Check sheet for the modelled part. Datum: model origin and axes. Units: mm. A direction names the side the tool comes from. Give positions to 0.01 mm unless a question says otherwise; leave off trailing zeros. Order: outer loops, then holes, each group sorted by start corner. A loop starts at its lowest first (then second) coordinate and runs counter-clockwise, first axis right, second up. Notation, with made-up numbers: (-28.5, 88.25) -> (-19.5, 88.25) arc R32 ccw to (-19.5, 127.25) -> close; hole circle Ø8 at (-22, 42.5). An arc over 180 degrees is marked (long way). One line per question, with ' | ' between items.
Autodesk Inventor part; units mm, degrees
ref_plane "YZ Plane" through (0, 0, 0) normal (1, 0, 0) x (0, 1, 0)
ref_plane "XZ Plane" through (0, 0, 0) normal (0, 1, 0) x (-1, 0, 0)
ref_plane "XY Plane" through (0, 0, 0) normal (0, 0, 1) x (1, 0, 0)
sketch "草圖1" plane through (0, 0, 0) normal (0, 1, 0) x (-1, 0, 0)
  line L0 (12, 16.5) -> (-12, 16.5)
  line L1 (-12, -16.5) -> (12, -16.5)
  line L2 (12, -16.5) -> (12, 16.5)
  line L3 (6.1, 11.4) -> (-6.1, 11.4)
  line L4 (-6.1, 11.4) -> (-6.1, -11.4)
  line L5 (-6.1, -11.4) -> (6.1, -11.4)
  line L6 (6.1, -11.4) -> (6.1, 11.4)
  circle A0 centre (8.5, 13.7) radius 1.5
  line L7 (12, 6) -> (9, 6)
  line L8 (9, 6) -> (9, -6)
  line L9 (9, -6) -> (12, -6)
  line L10 (12, -6) -> (12, 6)
  line L11 (0, -23.1) -> (0, 23.1)
  line L12 (16.8, 0) -> (-16.8, 0)
  circle A1 centre (8.5, -13.7) radius 1.5
  circle A2 centre (-8.5, 13.7) radius 1.5
  line L13 (-12, 6) -> (-9, 6)
  line L14 (-9, 6) -> (-9, -6)
  line L15 (-9, -6) -> (-12, -6)
  circle A3 centre (-8.5, -13.7) radius 1.5
  line L16 (-12, 16.5) -> (-12, 6)
  line L17 (-12, -6) -> (-12, -16.5)
  point P0 (0, 0)
  dimension "d0" = 16.5
  dimension "d1" = 33
  dimension "d2" = 24
  dimension "d4" = 12.2
  dimension "d5" = 22.8
  dimension "d6" = 6.1
  dimension "d7" = 11.4
  dimension "d8" = 3
  dimension "d9" = 3.5
  dimension "d10" = 2.8
  dimension "d11" = 12
  dimension "d12" = 3
  dimension "d13" = 6
extrude "擠出1" add sketch "草圖1" along normal mid plane 3 contours L2 L7 L8 L12 L6 L3 L11 L0 | L11 L3 L4 L12 L14 L13 L16 L0 | L2 L1 L11 L5 L6 L12 L8 L9 | L4 L5 L11 L1 L17 L15 L14 L12
fillet "圓角1" radius 3 4 edges at (12, 0, 16.5) (-12, 0, 16.5) (-12, 0, -16.5) (12, 0, -16.5)
properties part number "板子7"
Q1. Section check A-A (x = -2.75). Enter the section's corners in (y, z).
Result sheet:
outline: (-1.5, -16.5) -> (1.5, -16.5) -> (1.5, -11.4) -> (-1.5, -11.4) -> close; (-1.5, 11.4) -> (1.5, 11.4) -> (1.5, 16.5) -> (-1.5, 16.5) -> close
Q2. Depth check by flat-ended pin: pin 1 Ø0.9 at (x, y) = (11, 0.5) entering from +Z; pin 2 Ø1 at (y, z) = (0, 2) entering from -X; pin 3 Ø0.9 at (x, y) = (10.5, 0.5) entering from -Z. Enter the tip coordinate at first touch or a pass-through.
Result sheet:
pin 1: stops at z = 16.07 | pin 2: stops at x = -9 | pin 3: stops at z = -16.31
Q3. Section check B-B (z = -4). Enter the section's corners in (x, y), and give its area (3 significant figures).
Result sheet:
outline: (-9, -1.5) -> (-6.1, -1.5) -> (-6.1, 1.5) -> (-9, 1.5) -> close; (6.1, -1.5) -> (9, -1.5) -> (9, 1.5) -> (6.1, 1.5) -> close | area: 17.4 mm2
Q4. Thickness scan on line 1 (Z direction, x = 8.5, y = 0); line 2 (Z direction, x = -9.75, y = 0.4); line 3 (X direction, y = -0.75, z = -12.5). Record the ranges inside material, lowest first.
Result sheet:
line 1: z = -16.5 to -15.2, -12.2 to 12.2, 15.2 to 16.5 | line 2: z = -16.4 to -14.53, -12.87 to -6, 6 to 12.87, 14.53 to 16.4 | line 3: x = -12 to -9.4, -7.6 to 7.6, 9.4 to 12
Q5. Section check D-D (x = -8.5). Enter the section's corners in (y, z), and give its area (3 significant figures).
Result sheet:
outline: (-1.5, -16.5) -> (1.5, -16.5) -> (1.5, -15.2) -> (-1.5, -15.2) -> close; (-1.5, -12.2) -> (1.5, -12.2) -> (1.5, 12.2) -> (-1.5, 12.2) -> close; (-1.5, 15.2) -> (1.5, 15.2) -> (1.5, 16.5) -> (-1.5, 16.5) -> close | area: 81.0 mm2
Q6. Section check C-C (y = -0.95). Enter the section's corners in (x, z), and give its area (3 significant figures).
Result sheet:
outline: (-12, -13.5) arc R3 ccw to (-9, -16.5) -> (9, -16.5) arc R3 ccw to (12, -13.5) -> (12, -6) -> (9, -6) -> (9, 6) -> (12, 6) -> (12, 13.5) arc R3 ccw to (9, 16.5) -> (-9, 16.5) arc R3 ccw to (-12, 13.5) -> (-12, 6) -> (-9, 6) -> (-9, -6) -> (-12, -6) -> close; hole circle Ø3 at (-8.5, -13.7); hole circle Ø3 at (-8.5, 13.7); hole (-6.1, -11.4) -> (6.1, -11.4) -> (6.1, 11.4) -> (-6.1, 11.4) -> close; hole circle Ø3 at (8.5, -13.7); hole circle Ø3 at (8.5, 13.7) | area: 406 mm2
Q7. Access from +Z, -Z, +X, -X, +Y, -Y to the whole of each face (thin tool, end or side, straight path). Record for faces 4 (the face through (6.1, 0, 0)), 5 (the face through (10, 0, -6)), 6 (the face through (-9, 0, 0)).
Result sheet:
face 4: +Y, -Y | face 5: +X, +Y, -Y | face 6: -X, +Y, -Y
Q8. Mould release check, pull along Z, two halves, no side actions. Record for faces 1 (the face through (12, 0, 10)), 2 (the face through (-8.175, -0.021, 15.164)), 3 (the face through (11.1, 0.02, 15.64)): pulls with the +Z half, pulls with the -Z half, needs draft (parallel to the pull), parting line crosses it, or undercut.
Result sheet:
face 1: needs draft | face 2: undercut | face 3: pulls with the +Z half
